Study the drawing (mm; zero at the part's minimum x, y, z) and answer. Round coordinates to 2 decimals unless told otherwise and drop trailing zeros. Use one line per item in the form item = value.
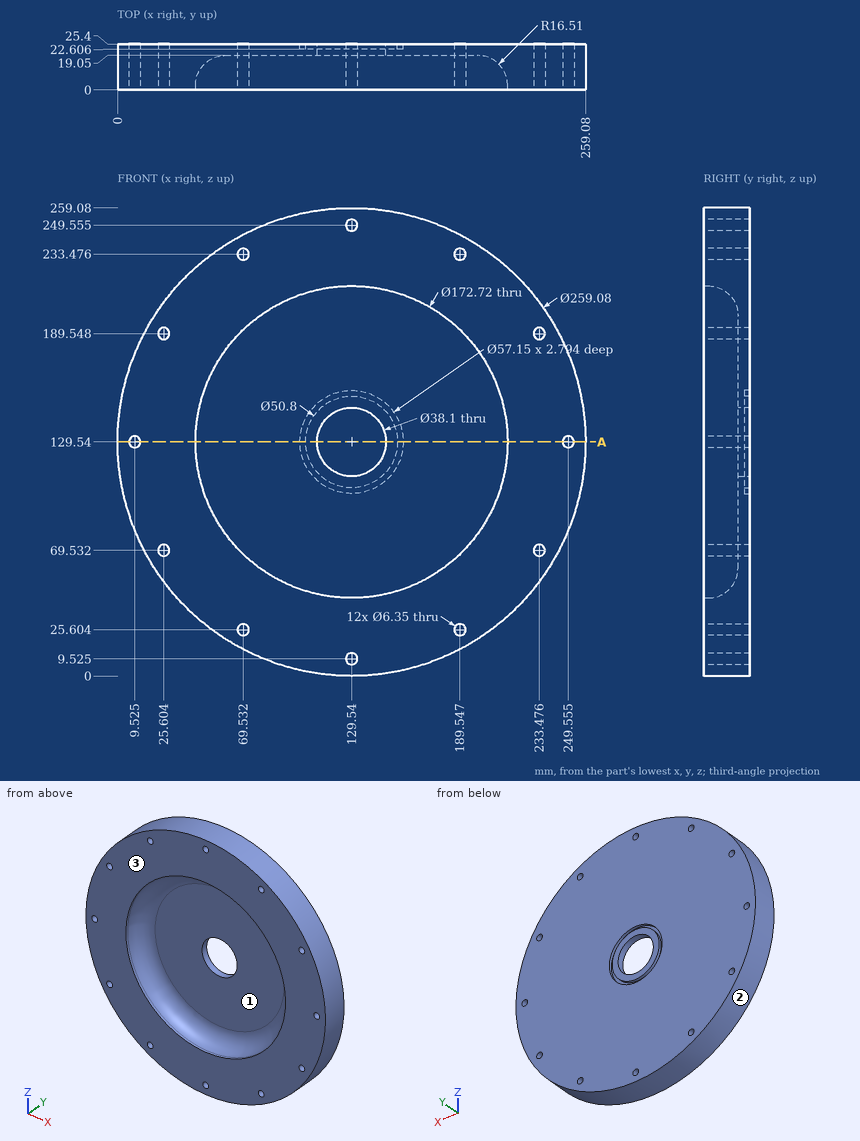
Item 1: Consider line 1 along Z through (x, y) = (129, 11.5) (1 decimal); line 2 along X through (y, z) = (0.8, 129.54); line 3 along Z through (x, y) = (67, 22.25) (1 decimal). Determine where each line is inside the solid, lowest interval first.
Findings:
line_1 = 0 to 6.4, 12.7 to 45.8, 213.3 to 246.4, 252.7 to 259.1
line_2 = 0 to 6.35, 12.7 to 43.18, 215.9 to 246.38, 252.73 to 259.08
line_3 = 16.1 to 23.7, 27.5 to 231.6, 235.4 to 243
Item 2: The part is cut by section A-A, the plane z = 129.54. Give the number of separate pieces and of enclosed holes in the cut face.
Findings:
separate_pieces = 4
enclosed_holes = 0
Item 3: Determine the mould class of the marked faces 1, 2 and 3 for opening direction X: released by +X, released by -X, zero draft, split by the parting line, or undercut.
Findings:
face_1 = undercut
face_2 = split by the parting line
face_3 = zero draft
Item 4: Flat-ended cylindrical pins translate along their axes: P1, Ø8.5, axis at x = 129.54, z = 9.525, coming from the -Y side; P2, Ø5, axis at x = 129.54, z = 249.555, coming from the +Y side; P3, Ø1, axis at x = 199.5, y = 21.5, coming from the -Z side; P4, Ø10, axis at y = 19, z = 75.5, coming from the -X side. Find the tip coordinate at first contact, or state that the pin passes through.
Findings:
P1 = 0
P2 = through
P3 = 20.2
P4 = 9.64
